The listing builds one solid part. Answer for the finished solid, in the listing's coordinates (mm). A direction names the side the tool comes from. Round coordinates to 2 decimals unless told otherwise and drop trailing zeros. Write each loop counter-clockwise with the first axis right and the second up, starting at its lowest first coordinate (ties: lowest second). Pieces come first, ordered by that corner, then holes. Notation, with made-up numbers: (45, 13.25) - (75, 13.25) arc R25 ccw to (75, 46.25) - close; hole circle Ø7 at (-14, 0). An arc over 180 degrees is marked (long way). Use a Markdown table: item, result. Add a question column.
1) A cutting plane is placed at C-C (x = 7.5). Give the vertices of the cut face in (y, z), then the cut area to 3 significant figures.
2) Find the intervals of material crossed by probe 1 along X at (y, z) = (0, -4.5); probe 2 along Z at (x, y) = (0, 2); probe 3 along Y at (x, z) = (-12, 1), in increasing order. Write a range as from..to.
3) A tool of negligible diameter and unlimited length cuts with its end or side. For faces 1 (the cylindrical face through (0, 2, -8)), 2 (the flat face through (0, 0, 25)), 3 (the cylindrical face through (9.44, 23.15, 12.32)), from which of +Z, -Z, +X, -X, +Y, -Y can it reach the whole face along a straight path? Write none if from no direction.
4) Determine the mould class of faces 4 (the flat face through (0, -6, 0)), 5 (the cylindrical face through (-17.755, -10.685, 12.325)) for opening direction Y: +Y half, -Y half, draft (parallel to the pull), parting line (faces both ways), or undercut.
5) A cutting plane is placed at A-A (z = 14.5). Give the vertices of the cut face in (x, y).
6) Each of these flat-tipped pins is pushed along its axis until it touches: P1, Ø2, axis at y = 3, z = 21, coming from the +X side; P2, Ø4, axis at x = 19, z = 15.5, coming from the -Y side; P3, Ø2.5, axis at x = 0, z = -7, coming from the +Y side. Where does it stop, or does it pass through?
7) A cutting plane is placed at B-B (y = -20). Give the vertices of the cut face in (x, z).
8) A cutting plane is placed at D-D (z = -5). Give the vertices of the cut face in (x, y).
```python
from build123d import *

# Parameters (mm, degrees)
SKETCH_1_R          = 30
EXTRUDE_1_DEPTH     = 25
EXTRUDE_5_DEPTH     = 10
CUT_EXTRUDE_1_REACH = 53.127
SKETCH_4_R          = 1
CUT_EXTRUDE_3_REACH = 51.244


with BuildPart() as part:
    # 草图1 → 凸台-拉伸1 (new body)
    with BuildSketch(Plane.XY):
        Circle(SKETCH_1_R)
    extrude(amount=EXTRUDE_1_DEPTH)

    # 草图2 → 凸台-拉伸5 (add)
    with BuildSketch(Plane.XY):
        with BuildLine():
            ThreePointArc((2.653299832, 1.4), (0, 3), (-2.653299832, 1.4))
            Line((-2.653299832, 1.4), (-1.428285686, 1.4))
            ThreePointArc((-1.428285686, 1.4), (0, 2), (1.428285686, 1.4))
            Line((1.428285686, 1.4), (2.653299832, 1.4))
        make_face()
        with BuildLine():
            Line((-1.428285686, 1.4), (-2.653299832, 1.4))
            ThreePointArc((-2.653299832, 1.4), (-0.721145097, -2.912035327), (3, 0))
            ThreePointArc((3, 0), (2.912035327, 0.721145097), (2.653299832, 1.4))
            Line((2.653299832, 1.4), (1.428285686, 1.4))
            ThreePointArc((1.428285686, 1.4), (1.851563039, 0.756117924), (2, 0))
            ThreePointArc((2, 0), (-0.756117924, -1.851563039), (-1.428285686, 1.4))
        make_face()
        with BuildLine():
            ThreePointArc((1.428285686, 1.4), (0, 2), (-1.428285686, 1.4))
            Line((-1.428285686, 1.4), (0, 1.4))
            Line((0, 1.4), (1.428285686, 1.4))
        make_face()
    extrude(amount=-EXTRUDE_5_DEPTH)

    # 草图4 → 切除-拉伸1 (cut, up to next)
    with BuildSketch(Plane(origin=(0, 3, 0), x_dir=(1, 0, 0), z_dir=(0, 1, 0)), mode=Mode.PRIVATE) as cut_extrude_1_sk1:
        with Locations(Location((0, 7, 0), (0, 0, 270))):
            Circle(SKETCH_4_R)
    cut_extrude_1_tool1 = extrude(cut_extrude_1_sk1.sketch, amount=-CUT_EXTRUDE_1_REACH, mode=Mode.PRIVATE) & part.part
    add(cut_extrude_1_tool1.solids().sort_by_distance((0, 3, -7))[0], mode=Mode.SUBTRACT)

    # 草图6 → 切除-拉伸3 (cut, up to next)
    with BuildSketch(Plane(origin=(0, 0, 0), x_dir=(-1, 0, 0), z_dir=(0, 0, -1)), mode=Mode.PRIVATE) as cut_extrude_3_sk1:
        with BuildLine():
            ThreePointArc((-10.60660171, 10.606601726), (-5.74025148, 13.85819299), (2e-09, 15))
            ThreePointArc((2e-09, 15), (5, 20.000000001), (0, 25))
            ThreePointArc((0, 25), (-9.567085809, 23.096988313), (-17.67766953, 17.67766953))
            ThreePointArc((-17.67766953, 17.67766953), (-17.677669526, 10.606601714), (-10.60660171, 10.606601726))
        make_face()
    cut_extrude_3_tool1 = extrude(cut_extrude_3_sk1.sketch, amount=-CUT_EXTRUDE_3_REACH, mode=Mode.PRIVATE) & part.part
    # 草图6 → 切除-拉伸3 (cut, up to next)
    with BuildSketch(Plane(origin=(0, 0, 0), x_dir=(-1, 0, 0), z_dir=(0, 0, -1)), mode=Mode.PRIVATE) as cut_extrude_3_sk2:
        with BuildLine():
            ThreePointArc((10.606601688, 10.606601748), (13.858192979, 5.740251505), (15, 0))
            ThreePointArc((15, 0), (20, -5), (25, 0))
            ThreePointArc((25, 0), (23.096988313, 9.567085809), (17.67766953, 17.67766953))
            ThreePointArc((17.67766953, 17.67766953), (10.606601733, 17.677669545), (10.606601688, 10.606601748))
        make_face()
    cut_extrude_3_tool2 = extrude(cut_extrude_3_sk2.sketch, amount=-CUT_EXTRUDE_3_REACH, mode=Mode.PRIVATE) & part.part
    # 草图6 → 切除-拉伸3 (cut, up to next)
    with BuildSketch(Plane(origin=(0, 0, 0), x_dir=(-1, 0, 0), z_dir=(0, 0, -1)), mode=Mode.PRIVATE) as cut_extrude_3_sk3:
        with BuildLine():
            ThreePointArc((-15, 0), (-19.999999994, 5), (-25, 1.2e-08))
            ThreePointArc((-25, 1.2e-08), (-23.096988305, -9.567085829), (-17.67766949, -17.677669569))
            ThreePointArc((-17.67766949, -17.677669569), (-10.606601708, -17.677669519), (-10.606601699, -10.606601737))
            ThreePointArc((-10.606601699, -10.606601737), (-13.858192983, -5.740251498), (-15, 0))
        make_face()
    cut_extrude_3_tool3 = extrude(cut_extrude_3_sk3.sketch, amount=-CUT_EXTRUDE_3_REACH, mode=Mode.PRIVATE) & part.part
    # 草图6 → 切除-拉伸3 (cut, up to next)
    with BuildSketch(Plane(origin=(0, 0, 0), x_dir=(-1, 0, 0), z_dir=(0, 0, -1)), mode=Mode.PRIVATE) as cut_extrude_3_sk4:
        with BuildLine():
            ThreePointArc((10.606601737, -10.606601699), (5.740251492, -13.858192985), (-1.3e-08, -15))
            ThreePointArc((-1.3e-08, -15), (-5, -19.999999976), (-6e-08, -25))
            ThreePointArc((-6e-08, -25), (9.567085826, -23.096988306), (17.677669598, -17.677669461))
            ThreePointArc((17.677669598, -17.677669461), (17.677669505, -10.606601693), (10.606601737, -10.606601699))
        make_face()
    cut_extrude_3_tool4 = extrude(cut_extrude_3_sk4.sketch, amount=-CUT_EXTRUDE_3_REACH, mode=Mode.PRIVATE) & part.part
    add(cut_extrude_3_tool1.solids().sort_by_distance((7.329332, 17.694573, 0))[0], mode=Mode.SUBTRACT)
    add(cut_extrude_3_tool2.solids().sort_by_distance((-17.694573, 7.329332, 0))[0], mode=Mode.SUBTRACT)
    add(cut_extrude_3_tool3.solids().sort_by_distance((17.694573, -7.329332, 0))[0], mode=Mode.SUBTRACT)
    add(cut_extrude_3_tool4.solids().sort_by_distance((-7.329332, -17.694573, 0))[0], mode=Mode.SUBTRACT)


solid = part.part
```
Entries:
| question | item | result |
|---|---|---|
| 1 | outline | (-29.05, 0) - (12.99, 0) - (12.99, 25) - (-29.05, 25) - close; (23.85, 0) - (29.05, 0) - (29.05, 25) - (23.85, 25) - close |
| 1 | area | 1,180 mm² |
| 2 | probe 1 | x = -3..-2, 2..3 |
| 2 | probe 2 | z = -10..-8, -6..25 |
| 2 | probe 3 | y = -27.5..-21.93, -9.62..9, 18.66..27.5 |
| 3 | face 1 | +Y |
| 3 | face 2 | +Z, +X, -X, +Y, -Y |
| 3 | face 3 | +Z, -Z |
| 4 | face 4 | draft |
| 4 | face 5 | undercut |
| 5 | outline | circle Ø60 at (0, 0); hole (-25, 0) arc R5 ccw to (-15, 0) arc R15 cw to (-10.61, 10.61) arc R5 ccw to (-17.68, 17.68) arc R25 ccw to start; hole (-17.68, -17.68) arc R25 ccw to (0, -25) arc R5 ccw to (0, -15) arc R15 cw to (-10.61, -10.61) arc R5 ccw to start; hole (0, 15) arc R15 cw to (10.61, 10.61) arc R5 ccw to (17.68, 17.68) arc R25 ccw to (0, 25) arc R5 ccw to start; hole (10.61, -10.61) arc R5 ccw to (17.68, -17.68) arc R25 ccw to (25, 0) arc R5 ccw to (15, 0) arc R15 cw to start |
| 6 | P1 | stops at x = 29.93 |
| 6 | P2 | stops at y = -24.72 |
| 6 | P3 | stops at y = 3 |
| 7 | outline | (-22.36, 0) - (-15, 0) - (-15, 25) - (-22.36, 25) - close; (5, 0) - (22.36, 0) - (22.36, 25) - (5, 25) - close |
| 8 | outline | circle Ø6 at (0, 0); hole (-1.43, 1.4) arc R2 ccw (long way) to (1.43, 1.4) - close |
